For this review, take the finished solid that the model builds, in its own axes (mm). Round coordinates to 2 decimals unless told otherwise and drop trailing zeros. Order: outer loops, then holes, each group sorted by start corner. A loop starts at its lowest first (then second) coordinate and runs counter-clockwise, first axis right, second up. Notation, with made-up numbers: (-21.5, -38.5) -> (5.5, -38.5) arc R20 cw to (5.5, -16.5) -> close; hole circle Ø8 at (10.25, 2). An arc over 180 degrees is marked (long way). Use a Markdown table: item, result. Add a question column.
1) Clearance check with flat-ended pins moving along their axes: P1, Ø0.6, axis at y = 0, z = -19, coming from the +X side; P2, Ø6, axis at x = -24.5, z = -25.5, coming from the -Y side; P3, Ø0.6, axis at x = 7.5, y = 0, coming from the -Z side. State where each tip first meets the part, or that it passes through.
2) Consider section A-A (y = 1.75). State the section outline as (x, z) points.
3) Wall thickness on line 1 along Z through (x, y) = (27.4, 1.5); line 2 along Z through (x, y) = (27.4, 0); line 3 along X through (y, z) = (3, -26.4): over which ranges is each line inside the solid? List them lowest first. Write a range as [from, to].
4) Consider section C-C (x = 16). State the section outline as (y, z) points, plus the area to 3 significant figures.
5) Consider section B-B (z = -22). State the section outline as (x, y) points.
```python
from build123d import *

# Parameters (mm, degrees)
SKETCH005_R      = 1.3
EXTRUDE003_DEPTH = 20
EXTRUDE039_DEPTH = 4
EXTRUDE042_DEPTH = 0.8
EXTRUDE002_DEPTH = 6
EXTRUDE037_DEPTH = 2


with BuildPart() as sweep001:
    # Sweep001: sweep along a path in Sketch034
    with BuildLine(Plane.XZ.offset(10)) as sweep001_path:
        Line((32, 12), (32, 26.4))
        ThreePointArc((32, 26.4), (30.652691, 29.652691), (27.4, 31))
        Line((27.4, 31), (-39.9, 31))
    # Sketch035 → Sweep001 (sweep)
    with BuildSketch(Plane.YZ):
        Polygon((5.3, 29.4), (3.7, 31), (3.7, 32), (6, 32), (6, 29.4), align=None)
    sweep(path=sweep001_path.line)


with BuildPart() as fusion030:
    # Sketch005 → Extrude003 (new body)
    with BuildSketch(Plane.XZ.offset(5)):
        with Locations((27.4, 26.4)):
            Circle(SKETCH005_R)
    extrude(amount=-EXTRUDE003_DEPTH)


with BuildPart() as fusion030_1:
    # Extrude003 placement: moved
    add(fusion030.part.moved(Location((0, -4, 0))))

    # Fusion030: union Sweep001
    add(sweep001.part)


with BuildPart() as top003:
    # Sketch028 → Extrude039 (new body)
    with BuildSketch(Plane.XZ.offset(10)):
        with BuildLine():
            ThreePointArc((32, 26.4), (30.652691, 29.652691), (27.4, 31))
            Line((27.4, 31), (-39.9, 31))
            Line((-39.9, 31), (-39.9, 29))
            Line((-39.9, 29), (27.4, 29))
            ThreePointArc((30, 26.4), (29.238478, 28.238478), (27.4, 29))
            Line((30, 12), (30, 26.4))
            Line((32, 12), (30, 12))
            Line((32, 26.4), (32, 12))
        make_face()
    extrude(amount=EXTRUDE039_DEPTH)


with BuildPart() as top003_1:
    # Extrude039 placement: moved
    add(top003.part.moved(Location((0, 14.5, 0))))


with BuildPart() as top002:
    # Sketch031 → Extrude042 (new body)
    with BuildSketch(Plane.XZ.offset(10)):
        with BuildLine():
            ThreePointArc((32, 26.4), (30.652691, 29.652691), (27.4, 31))
            Line((27.4, 31), (-39.9, 31))
            Line((-39.9, 31), (-39.9, 12))
            Line((-39.9, 12), (32, 12))
            Line((32, 26.4), (32, 12))
        make_face()
    extrude(amount=EXTRUDE042_DEPTH)


with BuildPart() as top002_1:
    # Extrude042 placement: moved
    add(top002.part.moved(Location((0, 15.3, 0))))


with BuildPart() as screw_hole_top:
    # Sketch004 → Extrude002 (new body)
    with BuildSketch(Plane.XZ.offset(10)):
        with BuildLine():
            ThreePointArc((25.36776, 29), (25.066548, 24.066548), (30, 24.36776))
            Line((30, 24.36776), (30, 26.4))
            ThreePointArc((30, 26.4), (29.238478, 28.238478), (27.4, 29))
            Line((25.36776, 29), (27.4, 29))
        make_face()
    extrude(amount=-EXTRUDE002_DEPTH)


with BuildPart() as screw_hole_top_1:
    # Extrude002 placement: moved
    add(screw_hole_top.part.moved(Location((0, 8.5, 0))))


with BuildPart() as top:
    # Sketch029 → Extrude037 (new body)
    with BuildSketch(Plane.XZ.offset(10)):
        with BuildLine():
            ThreePointArc((30.9, 26.4), (29.874874, 28.874874), (27.4, 29.9))
            Line((27.4, 29.9), (-22.5, 29.9))
            Line((-22.5, 29.9), (-22.5, 29))
            Line((-22.5, 29), (27.4, 29))
            ThreePointArc((30, 26.4), (29.238478, 28.238478), (27.4, 29))
            Line((30, 12), (30, 26.4))
            Line((30.9, 12), (30, 12))
            Line((30.9, 26.4), (30.9, 12))
        make_face()
    extrude(amount=EXTRUDE037_DEPTH)


with BuildPart() as top_1:
    # Extrude037 placement: moved
    add(top.part.moved(Location((0, 10.5, 0))))

    # Fusion028: union top003, top002, screw hole top
    add(top003_1.part)
    add(top002_1.part)
    add(screw_hole_top_1.part)

    # Cut024: cut Fusion030
    add(fusion030_1.part, mode=Mode.SUBTRACT)


with BuildPart() as part_mirroring001:
    # Part__Mirroring001: instance of top
    add(top_1.part.mirror(Plane(origin=(0, 0, 0), x_dir=(0, 1, 0), z_dir=(0, 0, 1))))


solid = part_mirroring001.part
```
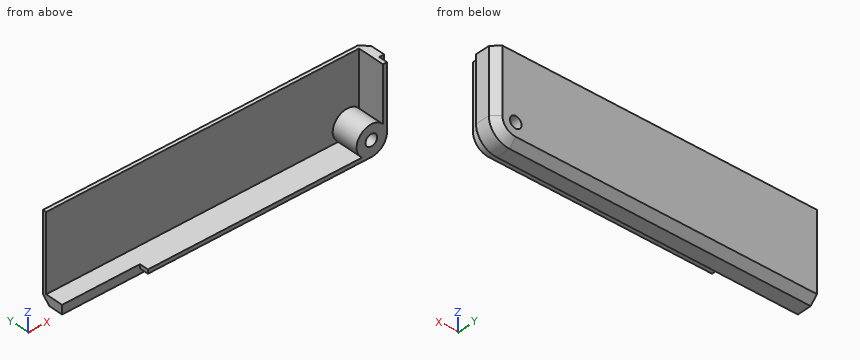
Results list:
| question | item | result |
|---|---|---|
| 1 | P1 | x = 30.9 |
| 1 | P2 | y = 4.5 |
| 1 | P3 | z = -29.9 |
| 2 | outline | (-39.9, -31) -> (27.4, -31) arc R4.6 ccw to (32, -26.4) -> (32, -12) -> (30, -12) -> (30, -24.37) arc R3.3 ccw (long way) to (25.37, -29) -> (-39.9, -29) -> close; hole circle Ø2.6 at (27.4, -26.4) |
| 3 | line 1 | [-31, -27.7], [-25.1, -23.1] |
| 3 | line 2 | [-29.9, -27.7], [-25.1, -23.1] |
| 3 | line 3 | [24.1, 26.1], [28.7, 32] |
| 4 | outline | (-1.5, -29.9) -> (0.5, -29.9) -> (0.5, -31) -> (3.7, -31) -> (5.3, -29.4) -> (5.3, -12) -> (4.5, -12) -> (4.5, -29) -> (-1.5, -29) -> close |
| 4 | area | 23.7 mm2 |
| 5 | outline | (-39.9, 4.5) -> (30, 4.5) -> (30, -1.5) -> (30.9, -1.5) -> (30.9, 0.5) -> (32, 0.5) -> (32, 3.7) -> (30.4, 5.3) -> (-39.9, 5.3) -> close |
